CAD build for the part. Positions are in the model's coordinates, mm. Face numbers are marked on the shaded views. A direction names the side the tool comes from. Give positions to 0.01 mm unless a question says otherwise; leave off trailing zeros. Order: outer loops, then holes, each group sorted by start corner. A loop starts at its lowest first (then second) coordinate and runs counter-clockwise, first axis right, second up.
Item 1: Wall check: L1, parallel to X at y = -27.5, z = 31; L2, parallel to X at y = -31, z = 69; L3, parallel to Z at x = -1, y = 4. Give the ranges that are in metal, low to high.
Item 2: Band-saw the part on B-B on x = 10.5. Give the cut face in (y, z).
Item 3: Band-saw the part on A-A on y = 11. Give the cut face in (x, z).
Item 4: Which spindle directions (+Z, -Z, +X, -X, +Y, -Y) get a long thin tool onto all of the face, cutting with end or side? Do the marked faces 5, 6, 7, 8 and 9. Say none if no direction does.
Item 5: Two-plate mould, pull along Z, no slides. Class the marked faces 1, 2, 3 and 4: released by +Z, released by -Z, zero draft, split by the parting line, or undercut.
Item 6: Band-saw the part on C-C on z = 61. Give the cut face in (x, y).
Item 7: Flat gauge pins, fed straight in: P1, Ø1.5, axis at x = -40.5, z = 38, coming from the -Y side; P2, Ø1.5, axis at y = -34.5, z = 44, coming from the -X side; P3, Ø10, axis at x = -37.5, z = 17, coming from the +Y side. Where does each tip first touch, or does it go through?
Item 8: Band-saw the part on D-D on y = -14. Give the cut face in (x, z), plus the area to 3 significant figures.
```python
from build123d import *

# Parameters (mm, degrees)
SKETCH3_W                         = 57.15
SKETCH3_H                         = 76.2
BOSS_EXTRUDE2_DEPTH               = 50.8
SKETCH4_W                         = 49.53
SKETCH4_H                         = 68.58
CUT_EXTRUDE2_DEPTH                = 44.45
CUT_EXTRUDE3_REACH                = 109.95
SKETCH5_W                         = 9.398
SKETCH5_H                         = 11.43
MOTOR_MOUNTING_SHAPE_DEPTH        = 57.15
MOTOR_MOUNTING_HOLES_REACH        = 131.428
SKETCH8_R                         = 1.6
SKETCH7_W                         = 7.62
SKETCH7_H                         = 29.66
TRAY_SUPPORT_MOUNTING_SHAPE_DEPTH = 44.45
SKETCH9_W                         = 15
SKETCH9_H                         = 15
BOSS_EXTRUDE3_DEPTH               = 66
SKETCH10_R                        = 3.175
CUT_EXTRUDE4_DEPTH                = 133.062873284
CHAMFER1_SIZE                     = 2
FILLET1_R                         = 2
CHAMFER2_SIZE                     = 1
CUT_EXTRUDE5_DEPTH                = 120.104586394


with BuildPart() as part:
    # Sketch3 → Boss-Extrude2 (new body)
    with BuildSketch(Plane(origin=(0, 0, 0), x_dir=(-1, 0, 0), z_dir=(0, 1, 0))):
        with Locations((28.575, 38.1)):
            Rectangle(SKETCH3_W, SKETCH3_H)
    extrude(amount=-BOSS_EXTRUDE2_DEPTH)

    # Sketch4 → Cut-Extrude2 (cut)
    with BuildSketch(Plane.XZ.offset(50.8)):
        with Locations((-28.575, 38.1)):
            Rectangle(SKETCH4_W, SKETCH4_H)
    extrude(amount=-CUT_EXTRUDE2_DEPTH, mode=Mode.SUBTRACT)

    # Sketch5 → Cut-Extrude3 (cut, up to next)
    with BuildSketch(Plane(origin=(-57.15, 0, 0), x_dir=(0, 0, -1), z_dir=(1, 0, 0)), mode=Mode.PRIVATE) as cut_extrude3_sk1:
        with Locations((-9.779, -41.275)):
            Rectangle(SKETCH5_W, SKETCH5_H)
    cut_extrude3_tool1 = extrude(cut_extrude3_sk1.sketch, amount=CUT_EXTRUDE3_REACH, mode=Mode.PRIVATE) & part.part
    add(cut_extrude3_tool1.solids().sort_by_distance((-57.15, -41.275, 9.779))[0], mode=Mode.SUBTRACT)

    # Sketch6 → Motor Mounting Shape (add)
    with BuildSketch(Plane.ZY.offset(57.15)):
        Polygon((46.54, 0), (46.54, 36.83), (0, 36.83), (0, 34.29), (44, 34.29), (44, 0), align=None)
    extrude(amount=-MOTOR_MOUNTING_SHAPE_DEPTH)

    # Sketch8 → Motor-Mounting-Holes (cut, up to next)
    with BuildSketch(Plane(origin=(0, 36.83, 0), x_dir=(1, 0, 0), z_dir=(0, 1, 0)), mode=Mode.PRIVATE) as motor_mounting_holes_sk1:
        with Locations(Location((-44.075, -7.77, 0), (0, 0, 270))):
            Circle(SKETCH8_R)
    motor_mounting_holes_tool1 = extrude(motor_mounting_holes_sk1.sketch, amount=-MOTOR_MOUNTING_HOLES_REACH, mode=Mode.PRIVATE) & part.part
    # Sketch8 → Motor-Mounting-Holes (cut, up to next)
    with BuildSketch(Plane(origin=(0, 36.83, 0), x_dir=(1, 0, 0), z_dir=(0, 1, 0)), mode=Mode.PRIVATE) as motor_mounting_holes_sk2:
        with Locations(Location((-13.075, -7.77, 0), (0, 0, 270))):
            Circle(SKETCH8_R)
    motor_mounting_holes_tool2 = extrude(motor_mounting_holes_sk2.sketch, amount=-MOTOR_MOUNTING_HOLES_REACH, mode=Mode.PRIVATE) & part.part
    # Sketch8 → Motor-Mounting-Holes (cut, up to next)
    with BuildSketch(Plane(origin=(0, 36.83, 0), x_dir=(1, 0, 0), z_dir=(0, 1, 0)), mode=Mode.PRIVATE) as motor_mounting_holes_sk3:
        with Locations(Location((-13.075, -38.77, 0), (0, 0, 270))):
            Circle(SKETCH8_R)
    motor_mounting_holes_tool3 = extrude(motor_mounting_holes_sk3.sketch, amount=-MOTOR_MOUNTING_HOLES_REACH, mode=Mode.PRIVATE) & part.part
    # Sketch8 → Motor-Mounting-Holes (cut, up to next)
    with BuildSketch(Plane(origin=(0, 36.83, 0), x_dir=(1, 0, 0), z_dir=(0, 1, 0)), mode=Mode.PRIVATE) as motor_mounting_holes_sk4:
        with Locations(Location((-44.075, -38.77, 0), (0, 0, 270))):
            Circle(SKETCH8_R)
    motor_mounting_holes_tool4 = extrude(motor_mounting_holes_sk4.sketch, amount=-MOTOR_MOUNTING_HOLES_REACH, mode=Mode.PRIVATE) & part.part
    # Sketch8 → Motor-Mounting-Holes (cut, up to next)
    with BuildSketch(Plane(origin=(0, 36.83, 0), x_dir=(1, 0, 0), z_dir=(0, 1, 0)), mode=Mode.PRIVATE) as motor_mounting_holes_sk5:
        with BuildLine():
            Line((-37.465, 0), (-19.685, 0))
            Line((-19.685, 0), (-19.685, -23.27))
            ThreePointArc((-19.685, -23.27), (-28.575, -32.16), (-37.465, -23.27))
            Line((-37.465, -23.27), (-37.465, 0))
        make_face()
    motor_mounting_holes_tool5 = extrude(motor_mounting_holes_sk5.sketch, amount=-MOTOR_MOUNTING_HOLES_REACH, mode=Mode.PRIVATE) & part.part
    add(motor_mounting_holes_tool1.solids().sort_by_distance((-44.075, 36.83, 7.77))[0], mode=Mode.SUBTRACT)
    add(motor_mounting_holes_tool2.solids().sort_by_distance((-13.075, 36.83, 7.77))[0], mode=Mode.SUBTRACT)
    add(motor_mounting_holes_tool3.solids().sort_by_distance((-13.075, 36.83, 38.77))[0], mode=Mode.SUBTRACT)
    add(motor_mounting_holes_tool4.solids().sort_by_distance((-44.075, 36.83, 38.77))[0], mode=Mode.SUBTRACT)
    add(motor_mounting_holes_tool5.solids().sort_by_distance((-28.575, 36.83, 15.191166))[0], mode=Mode.SUBTRACT)

    # Sketch7 → Tray Support Mounting Shape (add)
    with BuildSketch(Plane(origin=(0, 0, 0), x_dir=(1, 0, 0), z_dir=(0, 1, 0))):
        with Locations((-42.545, -61.37)):
            Rectangle(SKETCH7_W, SKETCH7_H)
        with Locations((-14.605, -61.37)):
            Rectangle(SKETCH7_W, SKETCH7_H)
    extrude(amount=TRAY_SUPPORT_MOUNTING_SHAPE_DEPTH)

    # Sketch9 → Boss-Extrude3 (add)
    # profile 1 of 2: a face of its own
    with BuildSketch(Plane.XZ.offset(50.8)):
        Polygon((0, 40), (-3.81, 40), (-3.81, 17), (0, 17), (19, 17), (19, 40), align=None)
        with Locations((7.5, 28.5)):
            Rectangle(SKETCH9_W, SKETCH9_H, mode=Mode.SUBTRACT)
    # profile 2 of 2: a face of its own
    with BuildSketch(Plane.XZ.offset(50.8)):
        Polygon((-53.34, 17), (-57.15, 17), (-76.15, 17), (-76.15, 40), (-57.15, 40), (-53.34, 40), align=None)
        with Locations((-64.65, 28.5)):
            Rectangle(SKETCH9_W, SKETCH9_H, mode=Mode.SUBTRACT)
    extrude(amount=-BOSS_EXTRUDE3_DEPTH)

    # Sketch10 → Cut-Extrude4 (cut, through all)
    with BuildSketch(Plane.ZY.offset(76.15)):
        with Locations((28.5, 4.2)):
            Circle(SKETCH10_R)
    extrude(amount=-CUT_EXTRUDE4_DEPTH, mode=Mode.SUBTRACT)

    # Chamfer1
    chamfer1_edges = [part.edges().sort_by_distance(p)[0] for p in [
        (0, 15.2, 28.5),
        (7.5, 15.2, 36),
        (15, 15.2, 28.5),
        (7.5, 15.2, 21),
        (-64.65, 15.2, 36),
        (-72.15, 15.2, 28.5),
        (-64.65, 15.2, 21),
        (-57.15, 15.2, 28.5),
    ]]
    chamfer(chamfer1_edges, length=CHAMFER1_SIZE)

    # Fillet1
    fillet1_edges = [part.edges().sort_by_distance(p)[0] for p in [
        (19, -17.8, 17),
        (19, -17.8, 40),
        (-76.15, -17.8, 40),
        (-76.15, -17.8, 17),
    ]]
    fillet(fillet1_edges, radius=FILLET1_R)

    # Chamfer2
    chamfer2_edges = [part.edges().sort_by_distance(p)[0] for p in [
        (-57.15, 4.2, 25.325),
        (15, 4.2, 25.325),
        (0, 4.2, 25.325),
        (-3.81, 4.2, 25.325),
        (-53.34, 4.2, 25.325),
        (-72.15, 4.2, 25.325),
        (19, 4.2, 25.325),
        (-76.15, 4.2, 25.325),
    ]]
    chamfer(chamfer2_edges, length=CHAMFER2_SIZE)

    # Sketch11 → Cut-Extrude5 (cut, through all)
    with BuildSketch(Plane(origin=(0, 0, 0), x_dir=(0, 0, -1), z_dir=(1, 0, 0))):
        Polygon((-44, 0), (-44, 34.29), (0, 34.29), (0, 51.599341861), (-81.196180942, 51.599341861), (-81.196180942, 0), align=None)
    extrude(amount=-CUT_EXTRUDE5_DEPTH, mode=Mode.SUBTRACT)


solid = part.part
```
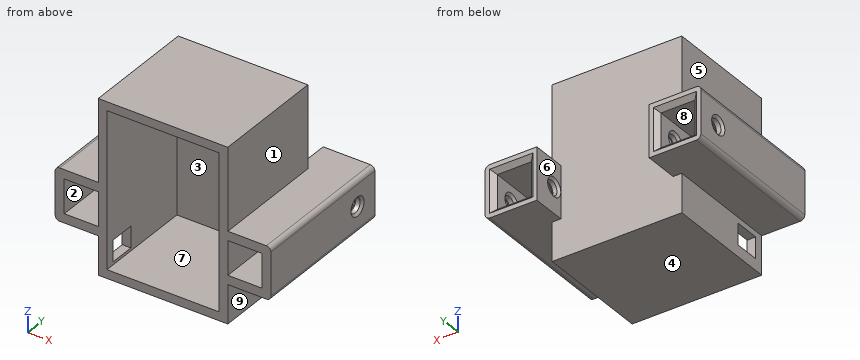
The answers:
1. L1: x = -76.15 to -72.15, -57.15 to -53.34, -3.81 to 0, 15 to 19
1. L2: x = -57.15 to -53.34, -3.81 to 0
1. L3: z = 17 to 25.33, 31.67 to 40
2. outline: (-50.8, 17) - (15.2, 17) - (15.2, 19) - (13.2, 21) - (-50.8, 21) - close; (-50.8, 36) - (13.2, 36) - (15.2, 38) - (15.2, 40) - (-50.8, 40) - close
3. outline: (-76.15, 19) arc R2 ccw to (-74.15, 17) - (-53.34, 17) - (-53.34, 40) - (-74.15, 40) arc R2 ccw to (-76.15, 38) - close; (-3.81, 17) - (17, 17) arc R2 ccw to (19, 19) - (19, 38) arc R2 ccw to (17, 40) - (-3.81, 40) - close; hole (-72.15, 21) - (-57.15, 21) - (-57.15, 36) - (-72.15, 36) - close; hole (0, 21) - (15, 21) - (15, 36) - (0, 36) - close
4. face 5: +Z, -X, +Y, -Y
4. face 6: +Z, -Z, +Y
4. face 7: -Y
4. face 8: +Y, -Y
4. face 9: -Z, +X, +Y, -Y
5. face 1: zero draft
5. face 2: undercut
5. face 3: undercut
5. face 4: released by -Z
6. outline: (-57.15, -50.8) - (-53.34, -50.8) - (-53.34, -6.35) - (-3.81, -6.35) - (-3.81, -50.8) - (0, -50.8) - (0, 0) - (-57.15, 0) - close
7. P1: stops at y = -6.35
7. P2: stops at x = -57.15
7. P3: stops at y = 0
8. outline: (-76.15, 19) arc R2 ccw to (-74.15, 17) - (-57.15, 17) - (-57.15, 0) - (0, 0) - (0, 17) - (17, 17) arc R2 ccw to (19, 19) - (19, 38) arc R2 ccw to (17, 40) - (0, 40) - (0, 76.2) - (-57.15, 76.2) - (-57.15, 40) - (-74.15, 40) arc R2 ccw to (-76.15, 38) - close; hole (-72.15, 21) - (-57.15, 21) - (-57.15, 36) - (-72.15, 36) - close; hole (-53.34, 3.81) - (-3.81, 3.81) - (-3.81, 72.39) - (-53.34, 72.39) - close; hole (0, 21) - (15, 21) - (15, 36) - (0, 36) - close
8. area: 1,380 mm2
